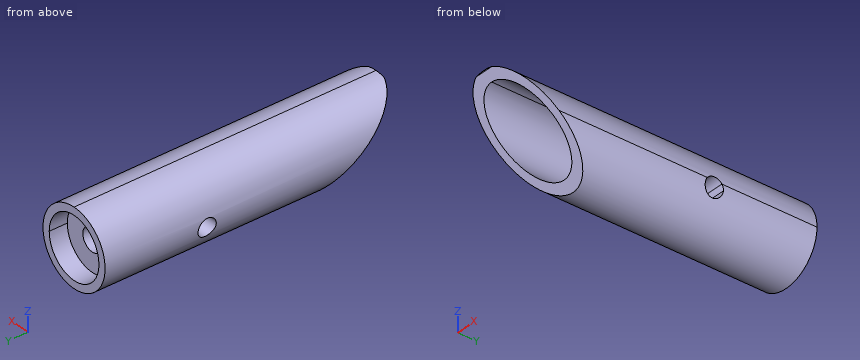
```python
from build123d import *

# Parameters (mm, degrees)
F1_DEPTH       = 127
F3_R           = 12.7
F4_DEPTH       = 40.005
F5_R           = 4.7625
F6_DEPTH       = 31.75
F8_DEPTH       = 25.4
F8_DEPTH_BACK  = 25.4
F10_DEPTH      = 25.4
F10_DEPTH_BACK = 25.4
F12_R          = 12.7
F13_DEPTH      = 7.62
F14_R          = 12.7


with BuildPart() as f1:
    # F0 (on Front) → F1 (new body)
    with BuildSketch(Plane.XZ):
        with BuildLine():
            ThreePointArc((0, 15.875), (-11.2253201513, -11.2253201513), (15.875, 0))
            ThreePointArc((15.875, 0), (11.2253201513, 11.2253201513), (0, 15.875))
        make_face()
        with BuildLine():
            ThreePointArc((12.7, 0), (-8.9802561211, -8.9802561211), (0, 12.7))
            ThreePointArc((0, 12.7), (8.9802561211, 8.9802561211), (12.7, 0))
        make_face(mode=Mode.SUBTRACT)
    extrude(amount=F1_DEPTH)

    # F3 (on offset) → F4 (join)
    with BuildSketch(Plane.XZ.offset(7.62)):
        Circle(F3_R)
    extrude(amount=F4_DEPTH)

    # F5 (on offset) → F6 (cut)
    with BuildSketch(Plane.XZ.offset(7.62)):
        Circle(F5_R)
    extrude(amount=F6_DEPTH, mode=Mode.SUBTRACT)

    # F7 (on Right) → F8 (cut, two sides)
    with BuildSketch(Plane.YZ) as f8_sk:
        Polygon((-89.1579282522, -16.1558650434), (-127.2579282522, 15.5941349566), (-127.2579282522, -16.1558650434), align=None)
    extrude(amount=-F8_DEPTH, mode=Mode.SUBTRACT)
    extrude(f8_sk.sketch, amount=F8_DEPTH_BACK, mode=Mode.SUBTRACT)

    # F9 (on Right) → F10 (cut, two sides)
    with BuildSketch(Plane.YZ) as f10_sk:
        with BuildLine():
            ThreePointArc((-39.9931731398, 0), (-46.6771131967, -3.4545031169), (-39.2481569672, -2.2631778847))
            ThreePointArc((-39.2481569672, -2.2631778847), (-39.4392007377, -1.0718526525), (-39.9931731398, 0))
        make_face()
    extrude(amount=-F10_DEPTH, mode=Mode.SUBTRACT)
    extrude(f10_sk.sketch, amount=F10_DEPTH_BACK, mode=Mode.SUBTRACT)

    # F12 (on offset) → F13 (join)
    with BuildSketch(Plane.XZ.offset(47.625)):
        Circle(F12_R)
    extrude(amount=F13_DEPTH)

    # F14
    f14_edges = [f1.edges().sort_by_distance(p)[0] for p in [
        (0, -55.245, -12.7),
    ]]
    fillet(f14_edges, radius=F14_R)


solid = f1.part
```
Verification items for the finished model (mm, model axes). Coordinates: 2 decimals unless noted, no trailing zeros. Loops run counter-clockwise (first coordinate to the right, second up) from the corner with the lowest first, then second, coordinate; pieces in that order, holes last. Notation, with made-up numbers: (-9.75, 55) -> (13.25, 55) arc R7 cw to (13.25, 59) -> close; hole circle Ø7 at (46, 38). An arc over 180 degrees is marked (long way). Answer in a Markdown table with one row per item. Add a question column.
1. Section check B-B, the plane y = -95. Enter the section's corners in (x, z) (3 decimals), then the cut area to 3 significant figures.
2. Depth check by flat-ended pin: P1, Ø8, axis at x = 4.5, y = -51, coming from the +Z side; P2, Ø1, axis at x = 9.5, y = -43.5, coming from the +Z side; P3, Ø6.5, axis at x = 0.5, z = 0.5, coming from the +Y side. Enter the tip coordinate at first touch or a pass-through.
3. Section check A-A, the plane x = 10. Enter the section's corners in (y, z) (3 decimals).
4. Section check C-C, the plane z = -10.5. Enter the section's corners in (x, y) (3 decimals), then the cut area to 3 significant figures.
5. Section check D-D, the plane y = -79. Enter the section's corners in (x, z) (3 decimals).
6. Material ranges on probe 1 along X at (y, z) = (-19, 0) (1 decimal); probe 2 along X at (y, z) = (-70.5, -9); probe 3 along Y at (x, z) = (5, -1), recorded low to high. Write a range as [from, to].
Derived:
| question | item | result |
|---|---|---|
| 1 | outline | (-11.163, -11.287) -> (-5.821, -11.287) arc R12.7 cw (long way) to (5.821, -11.287) -> (11.163, -11.287) arc R15.875 ccw (long way) to start |
| 1 | area | 226 mm² |
| 2 | P1 | stops at z = 15.87 |
| 2 | P2 | stops at z = 13.08 |
| 2 | P3 | stops at y = -39.37 |
| 3 | outline | (-123.34, 12.329) -> (-117.94, 7.829) -> (-67.945, 7.829) arc R7.829 cw to (-67.945, -7.829) -> (-99.15, -7.829) -> (-93.75, -12.329) -> (0, -12.329) -> (0, -7.829) -> (-7.62, -7.829) -> (-7.62, 7.829) -> (0, 7.829) -> (0, 12.329) -> close; hole circle Ø7.62 at (-43.058, -2.263) |
| 4 | outline | (-11.907, -95.945) -> (-7.144, -95.945) -> (-7.144, -67.945) arc R7.144 cw to (7.144, -67.945) -> (7.144, -95.945) -> (11.907, -95.945) -> (11.907, 0) -> (7.144, 0) -> (7.144, -7.62) -> (-7.144, -7.62) -> (-7.144, 0) -> (-11.907, 0) -> close |
| 4 | area | 1,700 mm² |
| 5 | outline | circle Ø31.75 at (0, 0); hole circle Ø25.4 at (0, 0) |
| 6 | probe 1 | x = [-15.9, -4.8], [4.8, 15.9] |
| 6 | probe 2 | x = [-13.08, -8.96], [8.96, 13.08] |
| 6 | probe 3 | y = [-56.31, -46.65], [-39.46, -7.62] |
